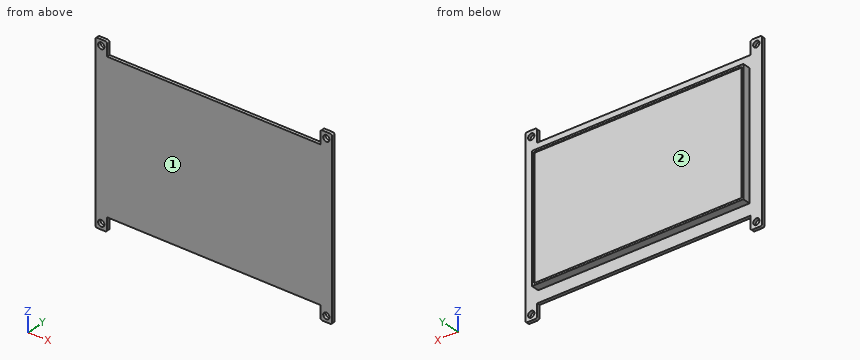
from build123d import *

# Parameters (mm, degrees)
SKETCH_1_R          = 1.6
EXTRUDE_1_DEPTH     = 1.6
SKETCH_2_W          = 108
SKETCH_2_H          = 64
EXTRUDE_2_DEPTH     = 4
SKETCH_3_W          = 106
SKETCH_3_H          = 62
CUT_EXTRUDE_1_DEPTH = 0.5


with BuildPart() as part:
    # 草图1 → 凸台-拉伸1 (new body)
    with BuildSketch(Plane(origin=(0, 0, 0), x_dir=(1, 0, 0), z_dir=(0, 1, 0))):
        with BuildLine():
            Line((54.5, 44), (54.5, 38))
            Line((54.5, 38), (-54.5, 38))
            Line((-54.5, 38), (-54.5, 44))
            ThreePointArc((-54.5, 44), (-54.792893219, 44.707106781), (-55.5, 45))
            Line((-55.5, 45), (-59.5, 45))
            ThreePointArc((-59.5, 45), (-60.207106781, 44.707106781), (-60.5, 44))
            Line((-60.5, 44), (-60.5, 38))
            Line((-60.5, 38), (-60.5, -38))
            Line((-60.5, -38), (-60.5, -44))
            ThreePointArc((-60.5, -44), (-60.207106781, -44.707106781), (-59.5, -45))
            Line((-59.5, -45), (-55.5, -45))
            ThreePointArc((-55.5, -45), (-54.792893219, -44.707106781), (-54.5, -44))
            Line((-54.5, -44), (-54.5, -38))
            Line((-54.5, -38), (54.5, -38))
            Line((54.5, -38), (54.5, -44))
            ThreePointArc((54.5, -44), (54.792893219, -44.707106781), (55.5, -45))
            Line((55.5, -45), (59.5, -45))
            ThreePointArc((59.5, -45), (60.207106781, -44.707106781), (60.5, -44))
            Line((60.5, -44), (60.5, 38))
            Line((60.5, 38), (60.5, 44))
            ThreePointArc((60.5, 44), (60.207106781, 44.707106781), (59.5, 45))
            Line((59.5, 45), (55.5, 45))
            ThreePointArc((55.5, 45), (54.792893219, 44.707106781), (54.5, 44))
        make_face()
        with Locations(Location((-57.5, -42, 0), (0, 0, 270))):
            Circle(SKETCH_1_R, mode=Mode.SUBTRACT)
        with Locations(Location((57.5, -42, 0), (0, 0, 270))):
            Circle(SKETCH_1_R, mode=Mode.SUBTRACT)
        with Locations(Location((-57.5, 42, 0), (0, 0, 270))):
            Circle(SKETCH_1_R, mode=Mode.SUBTRACT)
        with Locations(Location((57.5, 42, 0), (0, 0, 270))):
            Circle(SKETCH_1_R, mode=Mode.SUBTRACT)
    extrude(amount=EXTRUDE_1_DEPTH)

    # 草图2 → 凸台-拉伸2 (add)
    with BuildSketch(Plane(origin=(0, 1.6, 0), x_dir=(1, 0, 0), z_dir=(0, 1, 0))):
        Rectangle(SKETCH_2_W, SKETCH_2_H)
    extrude(amount=EXTRUDE_2_DEPTH)

    # 草图3 → 切除-拉伸1 (cut)
    with BuildSketch(Plane(origin=(0, 5.6, 0), x_dir=(1, 0, 0), z_dir=(0, 1, 0))):
        Rectangle(SKETCH_3_W, SKETCH_3_H)
    extrude(amount=-CUT_EXTRUDE_1_DEPTH, mode=Mode.SUBTRACT)


solid = part.part
Geometry check sheet. Reference: the model listing, model coordinates, mm. Face numbers are marked on the shaded views. Round coordinates to 2 decimals unless told otherwise and drop trailing zeros. Loops run counter-clockwise (first coordinate to the right, second up) from the corner with the lowest first, then second, coordinate; pieces in that order, holes last. Notation, with made-up numbers: (34.25, 43) -> (48.25, 43) arc R15 ccw to (48.25, 71) -> close; hole circle Ø5 at (49, 55.5). An arc over 180 degrees is marked (long way). Answer as a JSON object with one key per item and string values. Group by question number.
Item 1: Release check for a two-part mould opening along X. For the marked faces 1 and 2 record: pulls with the +X half, pulls with the -X half, needs draft (parallel to the pull), parting line crosses it, or undercut.
Item 2: Cross-section at A-A, the plane z = 42. Record the cut outline in (x, y), plus the area to 3 significant figures.
Item 3: Cross-section at D-D, the plane y = 3.85. Record the cut outline in (x, z).
Item 4: Cross-section at B-B, the plane x = 57.5. Record the cut outline in (y, z), plus the area to 3 significant figures.
Item 5: Depth check by flat-ended pin: pin 1 Ø1.2 at (y, z) = (4.5, 1) entering from +X; pin 2 Ø18.5 at (x, z) = (-19, -8.5) entering from +Y; pin 3 Ø3 at (x, y) = (-14.5, 3.5) entering from +Z; pin 4 Ø3 at (x, z) = (-57.5, 42) entering from -Y. Enter the tip coordinate at first touch or a pass-through.
Item 6: Cross-section at C-C, the plane z = -25. Record the cut outline in (x, y).
Item 7: Thickness scan on line 1 along X through (y, z) = (0.55, -42); line 2 along X through (y, z) = (4.4, 7); line 3 along Y through (x, z) = (-33, 8.5). Record the ranges inside material, lowest first.
Determined:
{
 "1": {"face 1": "needs draft", "face 2": "undercut"},
 "2": {"outline": "(-60.5, 0) -> (-59.1, 0) -> (-59.1, 1.6) -> (-60.5, 1.6) -> close; (-55.9, 0) -> (-54.5, 0) -> (-54.5, 1.6) -> (-55.9, 1.6) -> close; (54.5, 0) -> (55.9, 0) -> (55.9, 1.6) -> (54.5, 1.6) -> close; (59.1, 0) -> (60.5, 0) -> (60.5, 1.6) -> (59.1, 1.6) -> close", "area": "8.96 mm²"},
 "3": {"outline": "(-54, -32) -> (54, -32) -> (54, 32) -> (-54, 32) -> close"},
 "4": {"outline": "(0, -45) -> (1.6, -45) -> (1.6, -43.6) -> (0, -43.6) -> close; (0, -40.4) -> (1.6, -40.4) -> (1.6, 40.4) -> (0, 40.4) -> close; (0, 43.6) -> (1.6, 43.6) -> (1.6, 45) -> (0, 45) -> close", "area": "134 mm²"},
 "5": {"pin 1": "stops at x = 54", "pin 2": "stops at y = 5.1", "pin 3": "stops at z = 32", "pin 4": "passes through"},
 "6": {"outline": "(-60.5, 0) -> (60.5, 0) -> (60.5, 1.6) -> (54, 1.6) -> (54, 5.6) -> (53, 5.6) -> (53, 5.1) -> (-53, 5.1) -> (-53, 5.6) -> (-54, 5.6) -> (-54, 1.6) -> (-60.5, 1.6) -> close"},
 "7": {"line 1": "x = -60.5 to -59.1, -55.9 to -54.5, 54.5 to 55.9, 59.1 to 60.5", "line 2": "x = -54 to 54", "line 3": "y = 0 to 5.1"}
}
